```python
from build123d import *

# Parameters (mm, degrees)
SKETCH1_R   = 3.175
SKETCH1_R_2 = 2.16


with BuildPart() as part:
    # Sweep1: sweep along a path in Sketch2
    with BuildLine(Plane.XY) as sweep1_path:
        Line((-42.571045256, 93.062008577), (-20.574, 105.762008577))
        ThreePointArc((-20.574, 105.762008577), (-6.858, 105.762008577), (0, 93.883604139))
        Line((0, 93.883604139), (0, 0))
    # Sketch1 → Sweep1 (sweep)
    with BuildSketch(Plane(origin=(0, 0, 0), x_dir=(1, 0, 0), z_dir=(0, 1, 0))):
        Circle(SKETCH1_R)
        Circle(SKETCH1_R_2, mode=Mode.SUBTRACT)
    sweep(path=sweep1_path.line)


solid = part.part
```
Geometry: final body of the model. Coordinates: model frame, mm. A direction names the side the tool comes from. Round coordinates to 2 decimals unless told otherwise and drop trailing zeros. Write each loop counter-clockwise with the first axis right and the second up, starting at its lowest first coordinate (ties: lowest second). Pieces come first, ordered by that corner, then holes. Notation, with made-up numbers: (81, 52) -> (126, 52) arc R27 cw to (126, 82) -> close; hole circle Ø8 at (84, -5.5). An arc over 180 degrees is marked (long way). Return JSON: item names as keys, results as strings.
Q1. Section B-B on z = 0. Return the cut outline in (x, y) (1 decimal), and give its area (3 significant figures).
From the geometry:
{"outline": "(-44.2, 95.8) -> (-43.7, 94.9) -> (-21.7, 107.6) arc R15.9 cw to (2.2, 93.9) -> (2.2, 0) -> (3.2, 0) -> (3.2, 93.9) arc R16.9 ccw to (-22.2, 108.5) -> close; (-41.5, 91.2) -> (-41, 90.3) -> (-19, 103) arc R10.5 cw to (-3.2, 93.9) -> (-3.2, 0) -> (-2.2, 0) -> (-2.2, 93.9) arc R11.6 ccw to (-19.5, 103.9) -> close", "area": "300 mm2"}
Q2. Set-up query: faces 1 (the cylindrical face through (2.06, 46.28, 0.65)), 2 (the cylindrical face through (-32.449, 101.285, 0.649)). Return all of +Z, -Z, +X, -X, +Y, -Y with unobstructed straight access to the full face (end or side cutting, diameter ignored); none if empty.
From the geometry:
{"face 1": "-Y", "face 2": "none"}
Q3. Ray query, line 1 (X direction, y = 38, z = 0) (3 decimals); line 2 (Y direction, x = -18.5, z = 0.5). Return the intervals inside material, ascending.
From the geometry:
{"line 1": "-3.175 to -2.16, 2.16 to 3.175", "line 2": "103.32 to 104.47, 108.96 to 110.04"}
Q4. First-contact query: pin 1 Ø2 at (y, z) = (64.5, 0.5) entering from -X (3 decimals); pin 2 Ø6 at (x, y) = (-38.5, 90) entering from +Z; pin 3 Ø1 at (y, z) = (77, 1) entering from -X; pin 4 Ø2 at (y, z) = (48.5, 1) entering from +X (3 decimals). Flat tips, straight axial feed; report the tip coordinate or a pass-through.
From the geometry:
{"pin 1": "x = -3.175", "pin 2": "z = 2.69", "pin 3": "x = -3.14", "pin 4": "x = 3.175"}
Q5. Section A-A on y = 28.5. Return the cut outline in (x, z) (3 decimals).
From the geometry:
{"outline": "circle Ø6.35 at (0, 0); hole circle Ø4.32 at (0, 0)"}
